```python
from build123d import *

# Parameters (mm, degrees)
SKETCH080_W     = 75.5
SKETCH080_H     = 44
PAD043_DEPTH    = 1
SKETCH081_W     = 15
SKETCH081_H     = 44
PAD044_DEPTH    = 11
SKETCH082_W     = 18
SKETCH082_H     = 44
PAD045_DEPTH    = 1
SKETCH083_W     = 10.5
SKETCH083_H     = 39.5
PAD046_DEPTH    = 30.5
SKETCH084_W     = 7
SKETCH084_H     = 30
POCKET029_DEPTH = 41
SKETCH085_W     = 15
SKETCH085_H     = 6
POCKET030_DEPTH = 15
FILLET012_R     = 7.5
CHAMFER047_SIZE = 0.5
CHAMFER048_SIZE = 0.3


with BuildPart() as part:
    # Sketch080 → Pad043 (new body)
    with BuildSketch(Plane.XY):
        with Locations((-30.25, 0)):
            Rectangle(SKETCH080_W, SKETCH080_H)
    extrude(amount=-PAD043_DEPTH)

    # Sketch081 (on Face5 of Pad043) → Pad044 (join)
    with BuildSketch(Plane.XY):
        Rectangle(SKETCH081_W, SKETCH081_H)
    extrude(amount=PAD044_DEPTH)

    # Sketch082 (on Face5 of Pad044) → Pad045 (join)
    with BuildSketch(Plane.XY.offset(11)):
        with Locations((-1.5, 0)):
            Rectangle(SKETCH082_W, SKETCH082_H)
    extrude(amount=PAD045_DEPTH)

    # Sketch083 (on Face7 of Pad045) → Pad046 (join)
    with BuildSketch(Plane.XY.offset(12)):
        Rectangle(SKETCH083_W, SKETCH083_H)
    extrude(amount=PAD046_DEPTH)

    # Sketch084 (on Face15 of Pad046) → Pocket029 (cut)
    with BuildSketch(Plane.XY.offset(42.5)):
        Rectangle(SKETCH084_W, SKETCH084_H)
    extrude(amount=-POCKET029_DEPTH, mode=Mode.SUBTRACT)

    # Sketch085 (on Face6 of Pocket029) → Pocket030 (cut)
    with BuildSketch(Plane.YZ.offset(7.5)):
        with Locations((0, 4.5)):
            Rectangle(SKETCH085_W, SKETCH085_H)
    extrude(amount=-POCKET030_DEPTH, mode=Mode.SUBTRACT)

    # Fillet012
    fillet012_edges = [part.edges().sort_by_distance(p)[0] for p in [
        (0, -15, 1.5),
        (0, 15, 1.5),
    ]]
    fillet(fillet012_edges, radius=FILLET012_R)

    # Chamfer047
    chamfer047_edges = [part.edges().sort_by_distance(p)[0] for p in [
        (7.5, -22, 5.5),
        (7.5, 22, 5.5),
        (7.5, 0, 7.5),
        (7.5, -7.5, 4.5),
        (7.5, 0, 1.5),
        (7.5, 7.5, 4.5),
        (7.5, 0, -1),
        (-30.25, -22, -1),
        (-7.5, -22, 5.5),
        (-10.5, -22, 11.5),
        (-68, 0, -1),
        (-30.25, 22, -1),
        (-7.5, 22, 5.5),
        (-10.5, 22, 11.5),
        (-7.5, 0, 7.5),
        (-7.5, -7.5, 4.5),
        (-7.5, 0, 1.5),
        (-7.5, 7.5, 4.5),
    ]]
    chamfer(chamfer047_edges, length=CHAMFER047_SIZE)

    # Chamfer048
    chamfer048_edges = [part.edges().sort_by_distance(p)[0] for p in [
        (0, 19.75, 42.5),
        (-5.25, 0, 42.5),
        (5.25, 0, 42.5),
        (0, -19.75, 42.5),
        (-3.5, 0, 42.5),
        (0, -15, 42.5),
        (3.5, 0, 42.5),
        (0, 15, 42.5),
        (-5.25, -19.75, 27.25),
        (5.25, -19.75, 27.25),
        (-5.25, 19.75, 27.25),
        (5.25, 19.75, 27.25),
    ]]
    chamfer(chamfer048_edges, length=CHAMFER048_SIZE)


with BuildPart() as part_1:
    # Body015 placement: moved
    add(part.part.moved(Location((106.5, 75, -138))))


solid = part_1.part
```
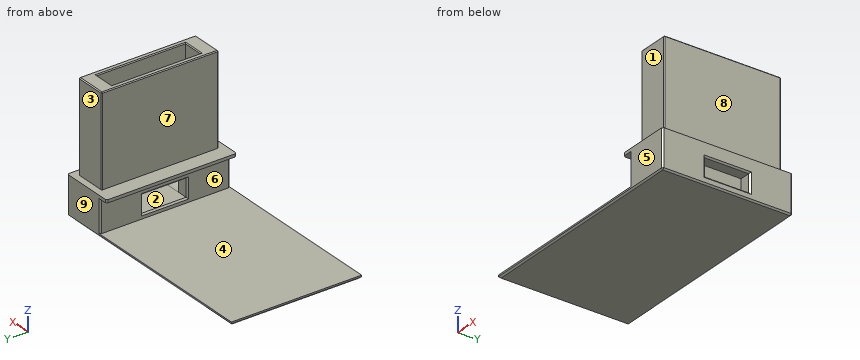
Source: CAD feature listing. Evaluate the final solid. Frame: model axes, mm. Face numbers are marked on the shaded views. A direction names the side the tool comes from. Give positions to 0.01 mm unless a question says otherwise; leave off trailing zeros. Order: outer loops, then holes, each group sorted by start corner. A loop starts at its lowest first (then second) coordinate and runs counter-clockwise, first axis right, second up.
(1) Contact query for flat-ended pins moving along their axis: P1, Ø8, axis at x = 76, y = 79, coming from the +Z side; P2, Ø4, axis at y = 67, z = -109, coming from the +X side; P3, Ø2, axis at x = 108, z = -112, coming from the +Y side; P4, Ø15.5, axis at x = 109, y = 72.5, coming from the +Z side. Output: stop coordinate, or through.
(2) Access query for the marked faces 5, 6, 7, 8 and 9. Directions: +Z, -Z, +X, -X, +Y, -Y. A direction counts if a zero-diameter tool reaches every point of the face in a straight line with its end or side. Return the directions, or none.
(3) Material intervals for line 1 along X through (y, z) = (73, -99); line 2 along X through (y, z) = (62, -129.5); line 3 along Z through (x, y) = (60, 71.5), sorted ascending.
(4) Section query B-B (y = 78.5). State how many separate pieces and enclosed holes the cut face has, plus the area to 3 significant figures.
(5) Section query D-D (y = 88). Return the cut outline in (x, z), plus the area to 3 significant figures.
(6) Pull-direction query (Y, two-part tool) for the marked faces 1, 2, 3 and 4; classes: +Y half, -Y half, draft (parallel to the pull), parting line (faces both ways), or undercut.
(7) Section query C-C (x = 66.5). Return the cut outline in (y, z), plus the area to 4 significant figures.
(8) Section query A-A (z = -106). Return the cut outline in (x, y), plus the area to 3 significant figures.
Outcome:
1. P1: stops at z = -138
1. P2: stops at x = 111.75
1. P3: stops at y = 94.75
1. P4: stops at z = -95.5
2. face 5: +Z, -Z, +X, -X, -Y
2. face 6: -X, +Y, -Y
2. face 7: +Z, -X, +Y, -Y
2. face 8: +Z, +X, +Y, -Y
2. face 9: +Z, -Z, +X, -X, +Y
3. line 1: x = 101.25 to 103, 110 to 111.75
3. line 2: x = 99 to 103, 110 to 114
3. line 3: z = -139 to -138
4. separate pieces: 3
4. enclosed holes: 0
4. area: 243 mm2
5. outline: (38.5, -138.5) - (39, -139) - (113.5, -139) - (114, -138.5) - (114, -126) - (111.75, -126) - (111.75, -95.8) - (111.45, -95.5) - (110.3, -95.5) - (110, -95.8) - (110, -134.1) - (103, -134.1) - (103, -95.8) - (102.7, -95.5) - (101.55, -95.5) - (101.25, -95.8) - (101.25, -126) - (96, -126) - (96, -127) - (99, -127) - (99, -138) - (38.5, -138) - close
5. area: 308 mm2
6. face 1: -Y half
6. face 2: undercut
6. face 3: +Y half
6. face 4: draft
7. outline: (53, -138.5) - (53.5, -139) - (96.5, -139) - (97, -138.5) - (97, -138) - (53, -138) - close
7. area: 43.75 mm2
8. outline: (101.25, 55.55) - (101.55, 55.25) - (111.45, 55.25) - (111.75, 55.55) - (111.75, 94.45) - (111.45, 94.75) - (101.55, 94.75) - (101.25, 94.45) - close; hole (103, 60) - (110, 60) - (110, 90) - (103, 90) - close
8. area: 205 mm2
